The drawing under review shows one solid part. Ordinate dimensions are in mm from its lowest x, y, z. Round coordinates to 2 decimals unless told otherwise and drop trailing zeros. Write each loop counter-clockwise with the first axis right and the second up, starting at its lowest first coordinate (ties: lowest second). Pieces come first, ordered by that corner, then holes. Notation, with made-up numbers: M -24,80 L 9,80 A18 ccw 9,90 Z; hole C -8.75,37 d8. An arc over 180 degrees is marked long. One line per item, written item: value. Start each with the question number.
1) Take a section at A-A, the plane y = 28. Write out the cut boundary in (x, z).
2) Take a section at C-C, the plane x = 29. Write out the cut boundary in (y, z).
3) Take a section at B-B, the plane x = 37.7. Write out the cut boundary in (y, z).
4) Take a section at D-D, the plane y = 14.3. Write out the cut boundary in (x, z), and give its area (3 significant figures).
5) Wall thickness on probe 1 along Y at (x, z) = (8.3, 1.7); probe 2 along Y at (x, z) = (43, 1.25); probe 3 along X at (y, z) = (24.5, 2.3): over which ranges is each line inside the solid? List them lowest first.
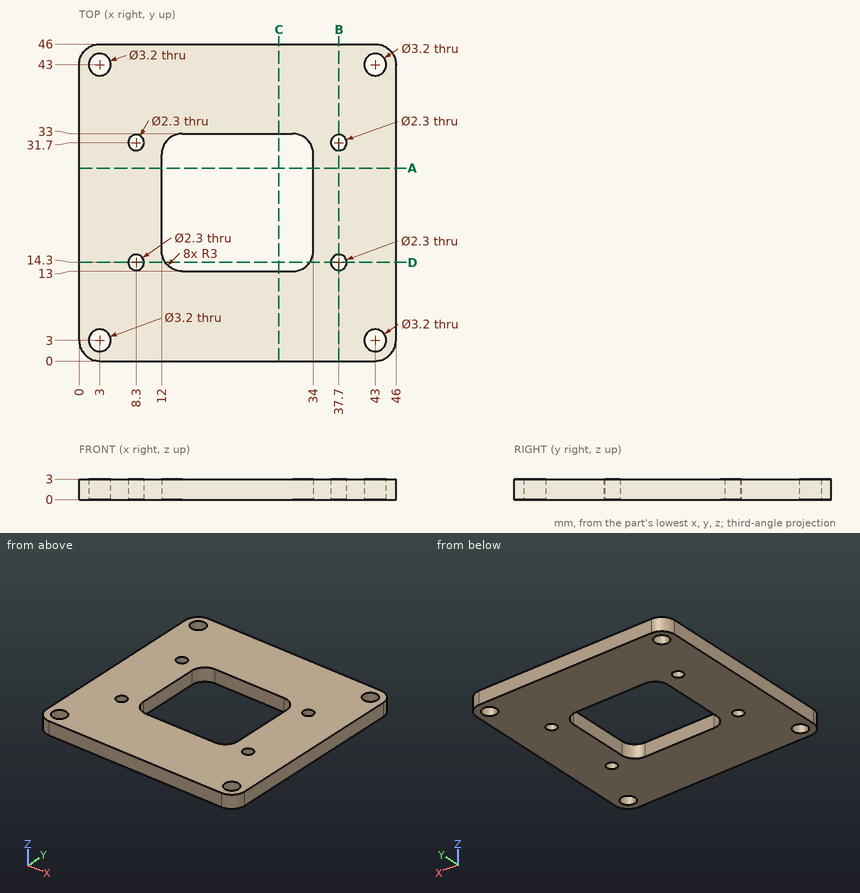
Checked values:
1. outline: M 0,0 L 12,0 L 12,3 L 0,3 Z; M 34,0 L 46,0 L 46,3 L 34,3 Z
2. outline: M 0,0 L 13,0 L 13,3 L 0,3 Z; M 33,0 L 46,0 L 46,3 L 33,3 Z
3. outline: M 0,0 L 13.15,0 L 13.15,3 L 0,3 Z; M 15.45,0 L 30.55,0 L 30.55,3 L 15.45,3 Z; M 32.85,0 L 46,0 L 46,3 L 32.85,3 Z
4. outline: M 0,0 L 7.15,0 L 7.15,3 L 0,3 Z; M 9.45,0 L 12.53,0 L 12.53,3 L 9.45,3 Z; M 33.47,0 L 36.55,0 L 36.55,3 L 33.47,3 Z; M 38.85,0 L 46,0 L 46,3 L 38.85,3 Z
4. area: 61.4 mm2
5. probe 1: y = 0 to 13.15, 15.45 to 30.55, 32.85 to 46
5. probe 2: y = 0 to 1.4, 4.6 to 41.4, 44.6 to 46
5. probe 3: x = 0 to 12, 34 to 46
